from build123d import *

# Parameters (mm, degrees)
SKETCH1_R           = 5
SKETCH1_R_2         = 1.5
EXTRUDE1_DEPTH      = 1.5
EXTRUDE2_DEPTH      = 8.228416147
EXTRUDE2_DEPTH_BACK = 8.228416147
SKETCH2_R           = 0.8
SKETCH3_R           = 0.8
EXTRUDE3_DEPTH      = 8.228416147


with BuildPart() as part:
    # Sketch1 → Extrude1 (new, symmetric)
    with BuildSketch(Plane.XY):
        Circle(SKETCH1_R)
        Circle(SKETCH1_R_2, mode=Mode.SUBTRACT)
    extrude(amount=EXTRUDE1_DEPTH, both=True)

    # Sketch2 → Extrude2 (cut, two sides: drawn at the far end of the back side and taken through both)
    with BuildSketch(Plane.XY.offset(-EXTRUDE2_DEPTH_BACK)):
        with Locations((-3.2, 0)):
            Circle(SKETCH2_R)
        with Locations((3.2, 0)):
            Circle(SKETCH2_R)
    extrude(amount=EXTRUDE2_DEPTH + EXTRUDE2_DEPTH_BACK, mode=Mode.SUBTRACT)

    # Sketch3 → Extrude3 (cut, through all)
    with BuildSketch(Plane(origin=(0, 0, 0), x_dir=(1, 0, 0), z_dir=(0, 1, 0))):
        with Locations(Location((0, 0, 0), (0, 0, 270))):
            Circle(SKETCH3_R)
    extrude(amount=-EXTRUDE3_DEPTH, mode=Mode.SUBTRACT)


solid = part.part
For this review, take the finished solid that the model builds, in its own axes (mm). Give positions to 0.01 mm unless a question says otherwise; leave off trailing zeros. Loops run counter-clockwise (first coordinate to the right, second up) from the corner with the lowest first, then second, coordinate; pieces in that order, holes last.
Item 1: Take a section at B-B, the plane y = 0. State the section outline as (x, z) points, and give its area (3 significant figures).
Item 2: Take a section at A-A, the plane x = 0. State the section outline as (y, z) points, and give its area (3 significant figures).
Item 3: Take a section at C-C, the plane x = 3.25. State the section outline as (y, z) points.
Item 4: Draft analysis for pull direction X (two halves, no side actions). For faces 1 (the flat face through (-1.2, 1.2, 1.5)), 2 (the cylindrical face through (-1.08, -4.88, 0.02)), 3 (the cylindrical face through (0, -3.1, -0.8)), 4 (the cylindrical face through (2.4, 0, 0)), state which applies: +X half, -X half, draft (parallel to the pull), parting line (faces both ways), or undercut.
Item 5: Take a section at D-D, the plane z = 0. State the section outline as (x, y) points, and give its area (3 significant figures).
Item 6: For line 1 along X through (y, z) = (0.25, 0.2); line 2 along Z through (x, y) = (0, -2.45); line 3 along X through (y, z) = (-3.25, 0.35), list the stretches that pass through material, from the lowest coordinate up.
Item 7: Insertion check: pin 1 (1 mm diameter, centred on y = 1, z = 1, fed in from -X); pin 2 (2.5 mm diameter, centred on x = 0, y = 0, fed in from -Z). Each pin has a flat end and moves straight along its axis. Give the tip position at first contact, or say it passes through.
Calculated:
1. outline: (-5, -1.5) - (-4, -1.5) - (-4, 1.5) - (-5, 1.5) - close; (-2.4, -1.5) - (-1.5, -1.5) - (-1.5, 1.5) - (-2.4, 1.5) - close; (1.5, -1.5) - (2.4, -1.5) - (2.4, 1.5) - (1.5, 1.5) - close; (4, -1.5) - (5, -1.5) - (5, 1.5) - (4, 1.5) - close
1. area: 11.4 mm2
2. outline: (-5, -1.5) - (-1.5, -1.5) - (-1.5, -0.8) - (-5, -0.8) - close; (-5, 0.8) - (-1.5, 0.8) - (-1.5, 1.5) - (-5, 1.5) - close; (1.5, -1.5) - (5, -1.5) - (5, 1.5) - (1.5, 1.5) - close
2. area: 15.4 mm2
3. outline: (-3.8, -1.5) - (-0.8, -1.5) - (-0.8, 1.5) - (-3.8, 1.5) - close; (0.8, -1.5) - (3.8, -1.5) - (3.8, 1.5) - (0.8, 1.5) - close
4. face 1: draft
4. face 2: parting line
4. face 3: undercut
4. face 4: undercut
5. outline: (-0.8, -4.94) - (-0.8, -1.27) arc R1.5 cw (long way) to (0.8, -1.27) - (0.8, -4.94) arc R5 ccw (long way) to start; hole circle Ø1.6 at (-3.2, 0); hole circle Ø1.6 at (3.2, 0)
5. area: 61.8 mm2
6. line 1: x = -4.99 to -3.96, -2.44 to -1.48, 1.48 to 2.44, 3.96 to 4.99
6. line 2: z = -1.5 to -0.8, 0.8 to 1.5
6. line 3: x = -3.8 to -0.72, 0.72 to 3.8
7. pin 1: stops at x = -4.97
7. pin 2: passes through
